Here's how the part is built. I have some questions about the finished solid (model axes, mm). Coordinates: 2 decimals unless noted, no trailing zeros. Loops run counter-clockwise (first coordinate to the right, second up) from the corner with the lowest first, then second, coordinate; pieces in that order, holes last.
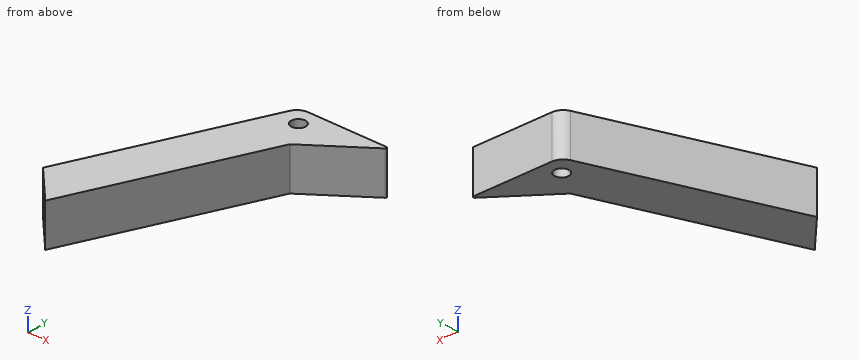
from build123d import *

# Parameters (mm, degrees)
F1_DEPTH = 15
F3_D     = 5.1


with BuildPart() as f1:
    # F0 (on Top) → F1 (new body)
    with BuildSketch(Plane.XY):
        with BuildLine():
            Line((16.345871, 27.436218), (-12.117236, 27.436218))
            ThreePointArc((-12.117236, 27.436218), (-14.649858, 26.655872), (-16.304115, 24.585473))
            Line((-16.304115, 24.585473), (-43.058704, -43.335009))
            Line((-43.058704, -43.335009), (-30.149364, -56.39547))
            Line((-30.149364, -56.39547), (-3.652537, 10.870645))
            ThreePointArc((-3.652537, 10.870645), (-3.586646, 10.988302), (-3.491709, 11.084071))
            Line((-3.491709, 11.084071), (16.650252, 26.539541))
            ThreePointArc((16.650252, 26.539541), (16.819336, 27.096937), (16.345871, 27.436218))
        make_face()
    extrude(amount=F1_DEPTH)

    # F3 (through all)
    with Locations(Plane.XY.offset(15)):
        with Locations((-9.721193, 20.991709)):
            Hole(F3_D / 2)


solid = f1.part
Q1. Will these pins go through, and if not, where does the flat tip stop? P1, Ø1.5, axis at y = -19.5, z = 10, coming from the +X side; P2, Ø4, axis at x = -33.5, z = 13, coming from the -Y side; P3, Ø2, axis at y = -47, z = 10.5, coming from the +X side.
Q2. Suppose I cut it at A-A on z = 1. Write out the boundary of the cut face in (x, y) (3 decimals).
Q3. Please list where these lines run through material, in increasing order: probe 1 along X at (y, z) = (-15, 4.25); probe 2 along X at (y, z) = (18, 12); probe 3 along Y at (x, z) = (8.5, 12.75).
Q4. Suppose I cut it at B-B on x = -27. Write out the boundary of the cut face in (y, z), and give its area (3 significant figures).
Q5. Suppose I cut it at C-C on y = 10. Write out the boundary of the cut face in (x, z).
Check values:
1. P1: stops at x = -15.32
1. P2: stops at y = -55.03
1. P3: stops at x = -26.05
2. outline: (-43.059, -43.335) - (-30.149, -56.395) - (-3.653, 10.871) arc R0.5 cw to (-3.492, 11.084) - (16.65, 26.54) arc R0.5 ccw to (16.346, 27.436) - (-12.117, 27.436) arc R4.5 ccw to (-16.304, 24.585) - close; hole circle Ø5.1 at (-9.721, 20.992)
3. probe 1: x = -31.9 to -13.84
3. probe 2: x = -18.9 to 5.52
3. probe 3: y = 20.29 to 27.44
4. outline: (-48.4, 0) - (-2.57, 0) - (-2.57, 15) - (-48.4, 15) - close
4. area: 687 mm2
5. outline: (-22.05, 0) - (-4, 0) - (-4, 15) - (-22.05, 15) - close
